from build123d import *

# Parameters (mm, degrees)
SKETCH1_R           = 80
SKETCH1_R_2         = 78.75
BOSS_EXTRUDE1_DEPTH = 20
SKETCH1_3_R         = 15.75
BOSS_EXTRUDE2_DEPTH = 20
SKETCH1_4_R         = 78.75
SKETCH1_4_R_2       = 15.75
BOSS_EXTRUDE3_DEPTH = 6


with BuildPart() as part:
    # Sketch1 → Boss-Extrude1 (new body)
    with BuildSketch(Plane(origin=(0, 0, 0), x_dir=(1, 0, 0), z_dir=(0, 1, 0))):
        with Locations(Location((0, 0, 0), (0, 0, 270))):
            Circle(SKETCH1_R)
        with Locations(Location((0, 0, 0), (0, 0, 270))):
            Circle(SKETCH1_R_2, mode=Mode.SUBTRACT)
    extrude(amount=BOSS_EXTRUDE1_DEPTH)



with BuildPart() as body_2:
    # Sketch1_3 → Boss-Extrude2 (new body)
    with BuildSketch(Plane(origin=(0, 0, 0), x_dir=(1, 0, 0), z_dir=(0, 1, 0))):
        with Locations(Location((0, 0, 0), (0, 0, 270))):
            Circle(SKETCH1_3_R)
    extrude(amount=BOSS_EXTRUDE2_DEPTH)


with BuildPart() as part_1:
    add(part.part)

    add(body_2.part)  # Boss-Extrude3 merges body 2
    # Sketch1_4 → Boss-Extrude3 (add)
    with BuildSketch(Plane(origin=(0, 0, 0), x_dir=(1, 0, 0), z_dir=(0, 1, 0))):
        with Locations(Location((0, 0, 0), (0, 0, 270))):
            Circle(SKETCH1_4_R)
        with Locations(Location((0, 0, 0), (0, 0, 270))):
            Circle(SKETCH1_4_R_2, mode=Mode.SUBTRACT)
    extrude(amount=BOSS_EXTRUDE3_DEPTH)


solid = part_1.part
The listing builds one solid part. Answer for the finished solid, in the listing's coordinates (mm). A direction names the side the tool comes from. Give positions to 0.01 mm unless a question says otherwise; leave off trailing zeros. Loops run counter-clockwise (first coordinate to the right, second up) from the corner with the lowest first, then second, coordinate; pieces in that order, holes last.
Item 1: Find the intervals of material crossed by line 1 along X through (y, z) = (15.75, 0); line 2 along Y through (x, z) = (-37, 30); line 3 along X through (y, z) = (19, -14.5), in increasing order.
Derived:
line 1: x = -80 to -78.75, -15.75 to 15.75, 78.75 to 80
line 2: y = 0 to 6
line 3: x = -78.67 to -77.4, -6.15 to 6.15, 77.4 to 78.67
Item 2: A cutting plane is placed at A-A (y = 14.5). Give the vertices of the cut face in (x, z), then the cut area to 3 significant figures.
Derived:
outline: circle Ø160 at (0, 0); circle Ø31.5 at (0, 0); hole circle Ø157.5 at (0, 0)
area: 1,400 mm2
Item 3: A cutting plane is placed at D-D (x = -39). Give the vertices of the cut face in (y, z), then the cut area to 3 significant figures.
Derived:
outline: (0, -69.85) - (20, -69.85) - (20, -68.41) - (6, -68.41) - (6, 68.41) - (20, 68.41) - (20, 69.85) - (0, 69.85) - close
area: 878 mm2
Item 4: Each of these flat-tipped pins is pushed along its axis until it touches: pin 1 Ø8 at (x, y) = (4, 11.5) entering from +Z; pin 2 Ø4 at (x, y) = (44.5, 2.5) entering from +Z; pin 3 Ø5 at (y, z) = (10, 26.5) entering from -X; pin 4 Ø1 at (x, y) = (-58.5, 9.5) entering from -Z. Where does it stop, or does it pass through?
Derived:
pin 1: stops at z = 80
pin 2: stops at z = 67.78
pin 3: stops at x = -76.32
pin 4: stops at z = -55.1
Item 5: Determine the mould class of faces 1 (the cylindrical face through (-78.1, 9.86, -17.34)), 2 (the cylindrical face through (15.616, 12.902, -2.05)), 3 (the flat face through (-53, 20, 59)) for opening direction Z: +Z half, -Z half, draft (parallel to the pull), parting line (faces both ways), or undercut.
Derived:
face 1: parting line
face 2: undercut
face 3: draft
Item 6: A cutting plane is placed at C-C (z = 0). Give the vertices of the cut face in (x, y).
Derived:
outline: (-80, 0) - (80, 0) - (80, 20) - (78.75, 20) - (78.75, 6) - (15.75, 6) - (15.75, 20) - (-15.75, 20) - (-15.75, 6) - (-78.75, 6) - (-78.75, 20) - (-80, 20) - close
Item 7: A tool of negligible diameter and unlimited length cuts with its end or side. For faces 4 (the cylindrical face through (-76.877, 12.902, -17.071)), 5 (the flat face through (0, 20, 0)), from which of +Z, -Z, +X, -X, +Y, -Y can it reach the whole face along a straight path? Write none if from no direction.
Derived:
face 4: +Y
face 5: +Z, -Z, +X, -X, +Y
Item 8: A cutting plane is placed at B-B (x = 0). Give the vertices of the cut face in (y, z), then the cut area to 3 significant figures.
Derived:
outline: (0, -80) - (20, -80) - (20, -78.75) - (6, -78.75) - (6, -15.75) - (20, -15.75) - (20, 15.75) - (6, 15.75) - (6, 78.75) - (20, 78.75) - (20, 80) - (0, 80) - close
area: 1,440 mm2
